The listing builds one solid part. Answer for the finished solid, in the listing's coordinates (mm). A direction names the side the tool comes from. Give positions to 0.01 mm unless a question says otherwise; leave off trailing zeros. Write each loop counter-clockwise with the first axis right and the second up, starting at its lowest first coordinate (ties: lowest second). Pieces come first, ordered by that corner, then holes. Notation, with made-up numbers: (17.5, -40) -> (57.5, -40) arc R15 ccw to (57.5, -24) -> close; hole circle Ø4 at (42, 76). An arc over 180 degrees is marked (long way). Use CSV: the item, a comma, the result in double quotes. Start each with the question number.
from build123d import *

# Parameters (mm, degrees)
SKETCH1_R           = 1.5
BOSS_EXTRUDE1_DEPTH = 5
SKETCH2_R           = 2
BOSS_EXTRUDE2_DEPTH = 11.45
BOSS_EXTRUDE6_DEPTH = 3.5
SKETCH4_R           = 0.5
BOSS_EXTRUDE5_DEPTH = 3.5
SKETCH5_W           = 3.014329637
SKETCH5_H           = 2.905175639
CUT_EXTRUDE1_DEPTH  = 19.229884569


with BuildPart() as part:
    # Sketch1 → Boss-Extrude1 (new body)
    with BuildSketch(Plane(origin=(0, 0, 0), x_dir=(1, 0, 0), z_dir=(0, 1, 0))):
        with Locations(Location((0, 0, 0), (0, 0, 270))):
            Circle(SKETCH1_R)
    extrude(amount=BOSS_EXTRUDE1_DEPTH)

    # Sketch2 → Boss-Extrude2 (add)
    with BuildSketch(Plane(origin=(0, 5, 0), x_dir=(1, 0, 0), z_dir=(0, 1, 0))):
        with Locations(Location((0, 0, 0), (0, 0, 270))):
            Circle(SKETCH2_R)
    extrude(amount=BOSS_EXTRUDE2_DEPTH)

    # Sketch6 → Boss-Extrude6 (add)
    with BuildSketch(Plane(origin=(0, 12.5, 0), x_dir=(1, 0, 0), z_dir=(0, 1, 0))):
        with BuildLine():
            Line((-2.524010645, -2.130146075), (-2.524010645, 3.851325134))
            ThreePointArc((-2.524010645, 3.851325134), (-2.231117427, 4.558431915), (-1.524010645, 4.851325134))
            Line((-1.524010645, 4.851325134), (-0.668009538, 4.851325134))
            ThreePointArc((-0.668009538, 4.851325134), (-0.399419742, 5.127808451), (-0.664387903, 5.407764478))
            Line((-0.664387903, 5.407764478), (-3.222291114, 5.531885865))
            Line((-3.222291114, 5.531885865), (-3.261907681, 5.966518704))
            Line((-3.261907681, 5.966518704), (-2.412173665, 6.135930219))
            Line((-2.412173665, 6.135930219), (-1.475989355, 6.135930219))
            ThreePointArc((-1.475989355, 6.135930219), (1.35243777, 4.964357344), (2.524010645, 2.135930219))
            Line((2.524010645, 2.135930219), (2.524010645, -3.851325134))
            ThreePointArc((2.524010645, -3.851325134), (2.231117427, -4.558431915), (1.524010645, -4.851325134))
            Line((1.524010645, -4.851325134), (0.668009538, -4.851325134))
            ThreePointArc((0.668009538, -4.851325134), (0.399419742, -5.127808451), (0.664387903, -5.407764478))
            Line((0.664387903, -5.407764478), (3.222291114, -5.531885865))
            Line((3.222291114, -5.531885865), (3.261907681, -5.966518704))
            Line((3.261907681, -5.966518704), (2.412173665, -6.135930219))
            Line((2.412173665, -6.135930219), (1.451593971, -6.130071682))
            ThreePointArc((1.451593971, -6.130071682), (-1.36104973, -4.949934938), (-2.524010645, -2.130146075))
        make_face()
    extrude(amount=BOSS_EXTRUDE6_DEPTH)

    # Sketch4 → Boss-Extrude5 (add)
    with BuildSketch(Plane(origin=(0, 12.5, 0), x_dir=(1, 0, 0), z_dir=(0, 1, 0))):
        with BuildLine():
            Line((0.882439523, -3.95958443), (1.971734047, 4.024950767))
            ThreePointArc((1.971734047, 4.024950767), (0.798204873, 5.569262908), (-0.746107269, 4.395733735))
            Line((-0.746107269, 4.395733735), (-1.835401792, -3.588801462))
            ThreePointArc((-1.835401792, -3.588801462), (-0.661872619, -5.133113604), (0.882439523, -3.95958443))
        make_face()
        with Locations((-0.476481135, -3.774192946)):
            Circle(SKETCH4_R, mode=Mode.SUBTRACT)
        with Locations((0.612813389, 4.210342251)):
            Circle(SKETCH4_R, mode=Mode.SUBTRACT)
    extrude(amount=BOSS_EXTRUDE5_DEPTH)

    # Sketch5 → Cut-Extrude1 (cut, through all)
    with BuildSketch(Plane(origin=(1.396633916, 0, 0.190536536), x_dir=(0.1351734199835011, 0, -0.9908219550100633), z_dir=(0.9908219550100633, 0, 0.1351734199835011))):
        with Locations((-4.25991475, 14.154353636)):
            Rectangle(SKETCH5_W, SKETCH5_H)
        with Locations((4.25991475, 14.154353636)):
            Rectangle(SKETCH5_W, SKETCH5_H)
    extrude(amount=-CUT_EXTRUDE1_DEPTH, mode=Mode.SUBTRACT)


solid = part.part
Q1. The mould has two halves that part along X. Classify faces 1 (the face through (2.382, 14.226, -3.191)), 2 (the face through (1, 14, 4.851)), 3 (the face through (-0.348, 14.134, -2.826)): +X half, -X half, draft (parallel to the pull), parting line (faces both ways), or undercut.
Q2. Section B-B on y = 3 is taken. Give the vertices of the cut face in (x, z), then the cut area to 3 significant figures.
Q3. Flat-ended cylindrical pins translate along their axes: pin 1 Ø3 at (x, z) = (-1, 4.5) entering from +Y; pin 2 Ø1.1 at (x, z) = (-0.5, -4.5) entering from -Y; pin 3 Ø1.5 at (x, y) = (1, 7) entering from -Z; pin 4 Ø1 at (y, z) = (3.5, 3) entering from +X. Find the tip coordinate at first contact, or state that the pin passes through.
Q4. Section A-A on z = 0 is taken. Give the vertices of the cut face in (x, y), then the cut area to 3 significant figures.
Q5. Straight lines are drawn through the part: L1, parallel to Y at x = 1.25, z = -3.75; L2, parallel to Y at x = 1, z = 4.5; L3, parallel to Y at x = -0.5, z = -1.5. For each, find the intervals that lie inside material, in ascending order.
Q6. For faces 4 (the face through (-2, 9, 0)), 5 (the face through (0.89, 14.17, 3.9)), 6 (the face through (-1.952, 16.222, -0.434)), 7 (the face through (0, 16.45, 0)), 8 (the face through (1.876, 14.175, -3.326)), determine the directions among +Z, -Z, +X, -X, +Y, -Y from which every point of the face is accessible in a straight line to the end or side of a thin tool.
Q7. Section C-C on y = 12 is taken. Give the vertices of the cut face in (x, z).
Output:
1,face 1,"+X half"
1,face 2,"draft"
1,face 3,"undercut"
2,outline,"circle Ø3 at (0, 0)"
2,area,"7.07 mm²"
3,pin 1,"y = 16"
3,pin 2,"y = 12.5"
3,pin 3,"z = -1.98"
3,pin 4,"through"
4,outline,"(-2.52, 12.5) -> (-2, 12.5) -> (-2, 5) -> (-1.5, 5) -> (-1.5, 0) -> (1.5, 0) -> (1.5, 5) -> (2, 5) -> (2, 12.5) -> (2.52, 12.5) -> (2.52, 16) -> (2, 16) -> (2, 16.45) -> (-2, 16.45) -> (-2, 16) -> (-2.52, 16) -> close"
4,area,"64.5 mm²"
5,L1,"12.5 to 12.7, 15.61 to 16"
5,L2,"12.5 to 16"
5,L3,"5 to 16.45"
6,face 4,"-Y"
6,face 5,"-X"
6,face 6,"+Y"
6,face 7,"+Z, -Z, +X, -X, +Y"
6,face 8,"-Z"
7,outline,"circle Ø4 at (0, 0)"
